from build123d import *

# Parameters (mm, degrees)
SKETCH_W     = 25.4
SKETCH_H     = 60
PAD_DEPTH    = 1.6
SKETCH001_W  = 8.3
SKETCH001_H  = 10.5
PAD001_DEPTH = 2.5
FILLET_R     = 1
SKETCH002_W  = 10
SKETCH002_H  = 8
PAD002_DEPTH = 2.5


with BuildPart() as part:
    # Sketch → Pad (new body)
    with BuildSketch(Plane.XY):
        with Locations((0, 30)):
            Rectangle(SKETCH_W, SKETCH_H)
    extrude(amount=PAD_DEPTH)

    # Sketch001 (on DatumPlane) → Pad001 (join)
    with BuildSketch(Plane.XY.offset(1.6)):
        with Locations((0, 3.25)):
            Rectangle(SKETCH001_W, SKETCH001_H)
    extrude(amount=PAD001_DEPTH)

    # Fillet
    fillet_edges = [part.edges().sort_by_distance(p)[0] for p in [
        (4.15, 3.25, 4.1),
        (-4.15, 3.25, 4.1),
        (-4.15, -1, 1.6),
        (4.15, -1, 1.6),
    ]]
    fillet(fillet_edges, radius=FILLET_R)

    # Sketch002 (on DatumPlane) → Pad002 (join)
    with BuildSketch(Plane.XY.offset(1.6)):
        with Locations((-9, 16)):
            Rectangle(SKETCH002_W, SKETCH002_H)
    extrude(amount=PAD002_DEPTH)


solid = part.part
The listing builds one solid part. Answer for the finished solid, in the listing's coordinates (mm). A direction names the side the tool comes from. Give positions to 0.01 mm unless a question says otherwise; leave off trailing zeros. Order: outer loops, then holes, each group sorted by start corner. A loop starts at its lowest first (then second) coordinate and runs counter-clockwise, first axis right, second up. Notation, with made-up numbers: (16, 47.25) - (29, 47.25) arc R20 ccw to (29, 86.25) - close; hole circle Ø5 at (39, 73.5). An arc over 180 degrees is marked (long way). One line per item, written item: value. Start each with the question number.
1) A cutting plane is placed at B-B on z = 0.65. Give the vertices of the cut face in (x, y).
2) Given pin 1 Ø3 at (x, y) = (-5, 23) entering from +Z; pin 2 Ø0.7 at (x, z) = (1.5, 3) entering from +Y; pin 3 Ø1.6 at (y, z) = (2.5, 2.5) entering from -X, each flat-ended and moving along its own axis, determine where each tip first touches the part or whether it passes through.
3) A cutting plane is placed at C-C on y = 35. Give the vertices of the cut face in (x, z), then the cut area to 3 significant figures.
4) Find the intervals of material crossed by L1, parallel to X at y = 18, z = 2.8; L2, parallel to Y at x = -10, z = 2.2; L3, parallel to X at y = 26.5, z = 0.8, in increasing order.
5) A cutting plane is placed at A-A on x = 2.5. Give the vertices of the cut face in (y, z).
6) A cutting plane is placed at D-D on x = -12. Give the vertices of the cut face in (y, z).
7) A tool of negligible diameter and unlimited length cuts with its end or side. For faces 4 (the face through (-4.15, 4, 2)), 5 (the face through (-4, 16, 3)), 6 (the face through (-9, 20, 3)), from which of +Z, -Z, +X, -X, +Y, -Y can it reach the whole face along a straight path? Write none if from no direction.
8) The mould has two halves that part along X. Classify faces 1 (the face through (-12.7, 30, 1)), 2 (the face through (12.7, 30, 1)), 3 (the face through (0, -1, 1.6)): released by +X, released by -X, zero draft, split by the parting line, or undercut.
Answer sheet:
1. outline: (-12.7, 0) - (12.7, 0) - (12.7, 60) - (-12.7, 60) - close
2. pin 1: stops at z = 1.6
2. pin 2: stops at y = 8.5
2. pin 3: stops at x = -4.15
3. outline: (-12.7, 0) - (12.7, 0) - (12.7, 1.6) - (-12.7, 1.6) - close
3. area: 40.6 mm2
4. L1: x = -14 to -4
4. L2: y = 12 to 20
4. L3: x = -12.7 to 12.7
5. outline: (-2, 1.6) - (0, 1.6) - (0, 0) - (60, 0) - (60, 1.6) - (8.5, 1.6) - (8.5, 4.1) - (-2, 4.1) - close
6. outline: (0, 0) - (60, 0) - (60, 1.6) - (20, 1.6) - (20, 4.1) - (12, 4.1) - (12, 1.6) - (0, 1.6) - close
7. face 4: +Z, -X, -Y
7. face 5: +Z, +X, +Y
7. face 6: +Z, +X, -X, +Y
8. face 1: released by -X
8. face 2: released by +X
8. face 3: zero draft
